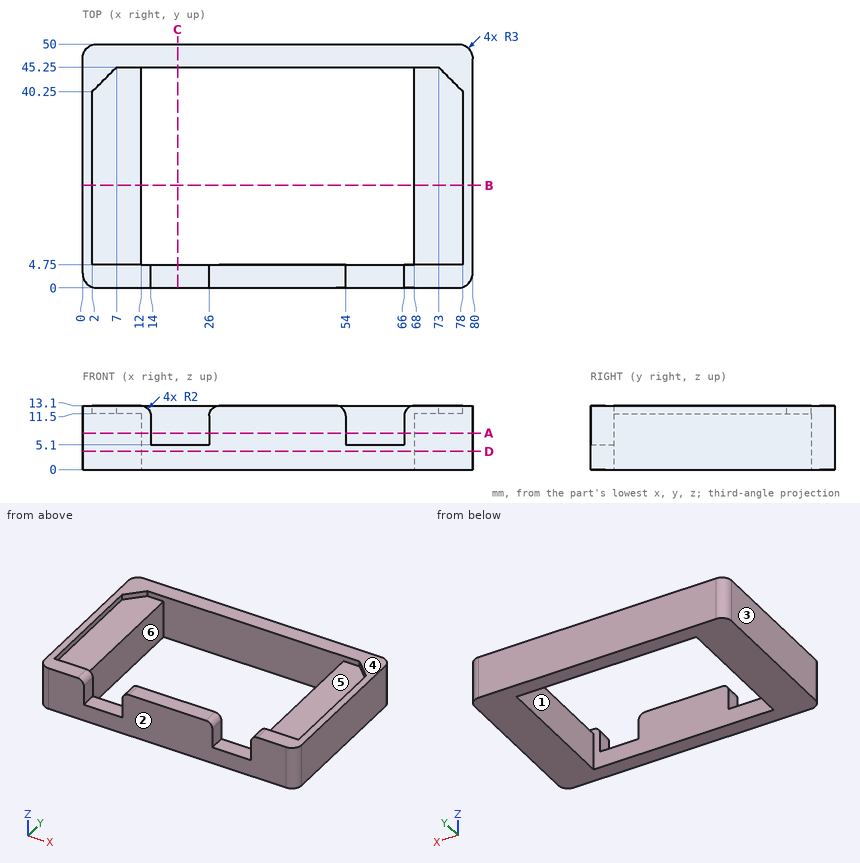
Part print with two shaded views. Sizes in mm from the minimum x, y, z corner. A direction names the side the tool comes from. Round coordinates to 2 decimals unless told otherwise and drop trailing zeros. Order: outer loops, then holes, each group sorted by start corner. A loop starts at its lowest first (then second) coordinate and runs counter-clockwise, first axis right, second up. Notation, with made-up numbers: M 43.5,82.25 L 83.5,82.25 A13 ccw 83.5,93.25 Z; hole C 2.25,-12.75 d2. An arc over 180 degrees is marked long. Answer in a Markdown table with one row per item. Add a question column.
Q1. Cut at C-C on x = 19.5. Give the cut face in (y, z), and give its area (4 significant figures).
Q2. Cut at A-A on z = 7.5. Give the cut face in (x, y), and give its area (3 significant figures).
Q3. Wall check: L1, parallel to Y at x = 36, z = 2; L2, parallel to X at y = 43, z = 1; L3, parallel to Y at x = 63, z = 10.5. Give the ranges that are in metal, low to high. Write a range as from..to.
Q4. Cut at D-D on z = 3.75. Give the cut face in (x, y), and give its area (3 significant figures).
Q5. 3-axis set-ups, long thin cutter, end or side, ignore diameter. For the marked faces 4, 5 and 6: which of +Z, -Z, +X, -X, +Y, -Y reach the whole face in a straight line?
Q6. Pin check, flat tips, straight feed: pin 1 (5 mm diameter, centred on x = 20.5, y = 2, fed in from +Z); pin 2 (3 mm diameter, centred on x = 74, y = 33, fed in from +Z). Stop position of each tip, or through.
Q7. Mould opens along X. For the marked faces 1, 2 and 3 say: +X half, -X half, draft (parallel to the pull), parting line (faces both ways), or undercut.
Q8. Cut at B-B on y = 21. Give the cut face in (x, z), and give its area (3 significant figures).
Established:
| question | item | result |
|---|---|---|
| 1 | outline | M 0,0 L 4.75,0 L 4.75,5.1 L 0,5.1 Z; M 45.25,0 L 50,0 L 50,13.1 L 45.25,13.1 Z |
| 1 | area | 86.45 mm2 |
| 2 | outline | M 0,3 A3 ccw 3,0 L 14,0 L 14,4.75 L 12,4.75 L 12,45.25 L 68,45.25 L 68,4.75 L 66,4.75 L 66,0 L 77,0 A3 ccw 80,3 L 80,47 A3 ccw 77,50 L 3,50 A3 ccw 0,47 Z; M 26,0 L 54,0 L 54,4.75 L 26,4.75 Z |
| 2 | area | 1,610 mm2 |
| 3 | L1 | y = 0..4.75, 45.25..50 |
| 3 | L2 | x = 0..12, 68..80 |
| 3 | L3 | y = 45.25..50 |
| 4 | outline | M 0,3 A3 ccw 3,0 L 77,0 A3 ccw 80,3 L 80,47 A3 ccw 77,50 L 3,50 A3 ccw 0,47 Z; hole M 12,4.75 L 68,4.75 L 68,45.25 L 12,45.25 Z |
| 4 | area | 1,720 mm2 |
| 5 | face 4 | +Z, +X, -X, +Y, -Y |
| 5 | face 5 | +Z |
| 5 | face 6 | +Z, -Z |
| 6 | pin 1 | stops at z = 5.1 |
| 6 | pin 2 | stops at z = 11.5 |
| 7 | face 1 | undercut |
| 7 | face 2 | draft |
| 7 | face 3 | -X half |
| 8 | outline | M 0,0 L 12,0 L 12,11.5 L 2,11.5 L 2,13.1 L 0,13.1 Z; M 68,0 L 80,0 L 80,13.1 L 78,13.1 L 78,11.5 L 68,11.5 Z |
| 8 | area | 282 mm2 |
